Read the model definition and answer for the solid it produces. Units are mm, in the model's axes. Round coordinates to 2 decimals unless told otherwise and drop trailing zeros. Order: outer loops, then holes, each group sorted by start corner. A loop starts at its lowest first (then second) coordinate and runs counter-clockwise, first axis right, second up. Notation, with made-up numbers: (-2.75, -17.5) - (7.25, -17.5) arc R12 ccw to (7.25, -2.5) - close; hole circle Ø11 at (53, -34.5). An arc over 180 degrees is marked (long way). Answer as a JSON object with one key per item and string values. Group by question number.
Q1. A cutting plane is placed at B-B on x = -22.5. Determine the outline of the cut face in (y, z).
Q2. A cutting plane is placed at D-D on x = 43. Determine the outline of the cut face in (y, z).
Q3. A cutting plane is placed at A-A on y = -13. Determine the outline of the cut face in (x, z), and give its area (3 significant figures).
Q4. Given pin 1 Ø1.9 at (x, z) = (-46, -4.5) entering from -Y; pin 2 Ø3 at (x, y) = (50, 13) entering from +Z; pin 3 Ø1.9 at (y, z) = (-29.5, -4.5) entering from +X; pin 4 Ø1.9 at (y, z) = (-30.5, -1.5) entering from -X, each flat-ended and moving along its own axis, determine where each tip first touches the part or whether it passes through.
Q5. Consider line 1 (X direction, y = -28.5, z = -3.25); line 2 (Y direction, x = 22.5, z = -2.5); line 3 (Y direction, x = 50, z = -1.25). Determine where each line is inside the solid, lowest interval first.
Q6. A cutting plane is placed at C-C on z = -4.5. Determine the outline of the cut face in (x, y), and give its area (3 significant figures).
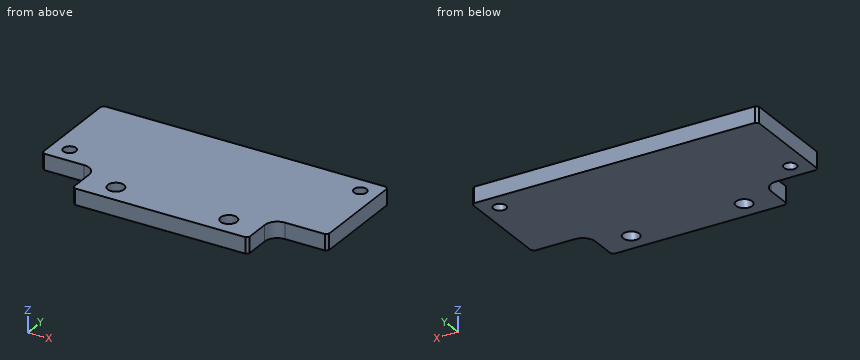
```python
from build123d import *

# Parameters (mm, degrees)
F0_R     = 3.25
F1_DEPTH = 6.35
F2_SIZE  = 1
F3_D     = 5


with BuildPart() as f1:
    # F0 (on Top) → F1 (new body)
    with BuildSketch(Plane.XY):
        with BuildLine():
            Line((57, -20), (57, 20))
            Line((57, 20), (-57, 20))
            Line((-57, 20), (-57, -20))
            Line((-57, -20), (-40, -20))
            ThreePointArc((-40, -20), (-36.4644660941, -21.4644660941), (-35, -25))
            Line((-35, -25), (-35, -36))
            Line((-35, -36), (35, -36))
            Line((35, -36), (35, -25))
            ThreePointArc((35, -25), (36.4644660941, -21.4644660941), (40, -20))
            Line((40, -20), (57, -20))
        make_face()
        with Locations((-22.5, -28)):
            Circle(F0_R, mode=Mode.SUBTRACT)
        with Locations((22.5, -28)):
            Circle(F0_R, mode=Mode.SUBTRACT)
    extrude(amount=-F1_DEPTH)

    # F2
    f2_edges = [f1.edges().sort_by_distance(p)[0] for p in [
        (-35, -36, -3.175),
        (-57, -20, -3.175),
        (35, -36, -3.175),
        (57, -20, -3.175),
        (-57, 20, -3.175),
        (57, 20, -3.175),
    ]]
    chamfer(f2_edges, length=F2_SIZE)

    # F3 (through all)
    with Locations(Plane.XY):
        with Locations((-50, -13), (50, 13)):
            Hole(F3_D / 2)


solid = f1.part
```
Result set:
{
 "1": {"outline": "(-36, -6.35) - (-31.25, -6.35) - (-31.25, 0) - (-36, 0) - close; (-24.75, -6.35) - (20, -6.35) - (20, 0) - (-24.75, 0) - close"},
 "2": {"outline": "(-20, -6.35) - (20, -6.35) - (20, 0) - (-20, 0) - close"},
 "3": {"outline": "(-57, -6.35) - (-52.5, -6.35) - (-52.5, 0) - (-57, 0) - close; (-47.5, -6.35) - (57, -6.35) - (57, 0) - (-47.5, 0) - close", "area": "692 mm²"},
 "4": {"pin 1": "stops at y = -20", "pin 2": "passes through", "pin 3": "stops at x = 35", "pin 4": "stops at x = -35"},
 "5": {"line 1": "x = -35 to -25.71, -19.29 to 19.29, 25.71 to 35", "line 2": "y = -36 to -31.25, -24.75 to 20", "line 3": "y = -20 to 10.5, 15.5 to 20"},
 "6": {"outline": "(-57, -19) - (-56, -20) - (-40, -20) arc R5 cw to (-35, -25) - (-35, -35) - (-34, -36) - (34, -36) - (35, -35) - (35, -25) arc R5 cw to (40, -20) - (56, -20) - (57, -19) - (57, 19) - (56, 20) - (-56, 20) - (-57, 19) - close; hole circle Ø5 at (-50, -13); hole circle Ø6.5 at (-22.5, -28); hole circle Ø6.5 at (22.5, -28); hole circle Ø5 at (50, 13)", "area": "5,580 mm²"}
}
